```python
from build123d import *

# Parameters (mm, degrees)
F0_W     = 96
F0_H     = 48
F1_DEPTH = 2
F2_W     = 96
F2_H     = 48
F2_W_2   = 9
F2_H_2   = 38
F3_DEPTH = 22
F0_W_2   = 110
F0_H_2   = 60
F4_DEPTH = 5
F5_R     = 4.99999
F6_SIZE  = 1.5


# Not quite as in the source:
# - a fillet or chamfer is up to 0.001 mm smaller than in the source, because OpenCascade refuses the exact size
# - a feature names something its author has since deleted; it is built from what else it names


with BuildPart() as f1:
    # F0 (on Top) → F1 (new body)
    with BuildSketch(Plane.XY):
        Rectangle(F0_W, F0_H)
    extrude(amount=F1_DEPTH)

    # F2 (on face) → F3 (join)
    with BuildSketch(Plane.XY.offset(2)):
        Rectangle(F2_W, F2_H)
        with Locations((-38.5, 0)):
            Rectangle(F2_W_2, F2_H_2, mode=Mode.SUBTRACT)
        with Locations((-23.1, 0)):
            Rectangle(F2_W_2, F2_H_2, mode=Mode.SUBTRACT)
        with Locations((-7.7, 0)):
            Rectangle(F2_W_2, F2_H_2, mode=Mode.SUBTRACT)
        with Locations((7.7, 0)):
            Rectangle(F2_W_2, F2_H_2, mode=Mode.SUBTRACT)
        with Locations((23.1, 0)):
            Rectangle(F2_W_2, F2_H_2, mode=Mode.SUBTRACT)
        with Locations((38.5, 0)):
            Rectangle(F2_W_2, F2_H_2, mode=Mode.SUBTRACT)
    extrude(amount=F3_DEPTH)

    # F0 (on Top) → F4 (join)
    with BuildSketch(Plane.XY):
        Rectangle(F0_W_2, F0_H_2)
        Rectangle(F0_W, F0_H, mode=Mode.SUBTRACT)
    extrude(amount=F4_DEPTH)

    # F5 (radius 5 in the source; OpenCascade refuses exactly that, so slightly less here)
    f5_edges = [f1.edges().sort_by_distance(p)[0] for p in [
        (0, -30, 5),
        (-55, 0, 5),
        (0, 30, 5),
        (55, 0, 5),
        (55, -30, 2.5),
        (55, 30, 2.5),
        (-55, -30, 2.5),
        (-55, 30, 2.5),
    ]]
    fillet(f5_edges, radius=F5_R)

    # F6
    f6_edges = [f1.edges().sort_by_distance(p)[0] for p in [
        (0, -24, 24),
        (-48, 0, 24),
        (0, 24, 24),
        (48, 0, 24),
        (-43, 0, 24),
        (-34, 0, 24),
        (-38.5, -19, 24),
        (-38.5, 19, 24),
        (-23.1, -19, 24),
        (-18.6, 0, 24),
        (-27.6, 0, 24),
        (-23.1, 19, 24),
        (-7.7, 19, 24),
        (-12.2, 0, 24),
        (-7.7, -19, 24),
        (-3.2, 0, 24),
        (3.2, 0, 24),
        (12.2, 0, 24),
        (7.7, -19, 24),
        (7.7, 19, 24),
        (18.6, 0, 24),
        (23.1, 19, 24),
        (27.6, 0, 24),
        (23.1, -19, 24),
        (38.5, -19, 24),
        (34, 0, 24),
        (43, 0, 24),
        (38.5, 19, 24),
    ]]
    chamfer(f6_edges, length=F6_SIZE)


solid = f1.part
```
Source: CAD feature listing. Evaluate the final solid. Frame: model axes, mm. A direction names the side the tool comes from. Give positions to 0.01 mm unless a question says otherwise; leave off trailing zeros. Order: outer loops, then holes, each group sorted by start corner. A loop starts at its lowest first (then second) coordinate and runs counter-clockwise, first axis right, second up.
(1) Material intervals for line 1 along Y through (x, z) = (-41, 12.5); line 2 along Z through (x, y) = (42.5, -14.5); line 3 along Y through (x, z) = (-31, 12.75), sorted ascending.
(2) Contact query for flat-ended pins moving along their axis: P1, Ø2, axis at x = -26, z = 2.5, coming from the -Y side; P2, Ø4.5, axis at x = -9, y = -5.5, coming from the +Z side; P3, Ø7, axis at x = -36.5, z = 17, coming from the +Y side. Output: stop coordinate, or through.
(3) Section query B-B (z = 12). Return the cut outline in (x, y).
(4) Pull-direction query (X, two-part tool) for faces 1 (the face through (18.6, 0, 12)), 2 (the face through (53, 0, 4)), 3 (the face through (-54, 0, 3)), 4 (the face through (-1, 0, 0)); classes: +X half, -X half, draft (parallel to the pull), parting line (faces both ways), or undercut.
(5) Access query for faces 5 (the face through (1, 29, 3)), 6 (the face through (3.2, 0, 12)), 7 (the face through (-1, -24, 14)). Directions: +Z, -Z, +X, -X, +Y, -Y. A direction counts if a zero-diameter tool reaches every point of the face in a straight line with its end or side. Return the directions, or none.
Outcome:
1. line 1: y = -24 to -19, 19 to 24
1. line 2: z = 0 to 2
1. line 3: y = -24 to 24
2. P1: stops at y = -29.77
2. P2: stops at z = 2
2. P3: stops at y = 24
3. outline: (-48, -24) - (48, -24) - (48, 24) - (-48, 24) - close; hole (-43, -19) - (-34, -19) - (-34, 19) - (-43, 19) - close; hole (-27.6, -19) - (-18.6, -19) - (-18.6, 19) - (-27.6, 19) - close; hole (-12.2, -19) - (-3.2, -19) - (-3.2, 19) - (-12.2, 19) - close; hole (3.2, -19) - (12.2, -19) - (12.2, 19) - (3.2, 19) - close; hole (18.6, -19) - (27.6, -19) - (27.6, 19) - (18.6, 19) - close; hole (34, -19) - (43, -19) - (43, 19) - (34, 19) - close
4. face 1: undercut
4. face 2: +X half
4. face 3: -X half
4. face 4: draft
5. face 5: +Z, +X, -X, +Y
5. face 6: +Z
5. face 7: +Z, +X, -X, -Y
